Build history of the part. All positions in model axes, mm. Give positions to 0.01 mm unless a question says otherwise; leave off trailing zeros. Order: outer loops, then holes, each group sorted by start corner. A loop starts at its lowest first (then second) coordinate and runs counter-clockwise, first axis right, second up. Notation, with made-up numbers: (49, 12.5) - (74, 12.5) arc R12 ccw to (74, 16.5) - close; hole circle Ø10 at (-27, 24.25). An arc over 180 degrees is marked (long way). One line per item, written item: value.
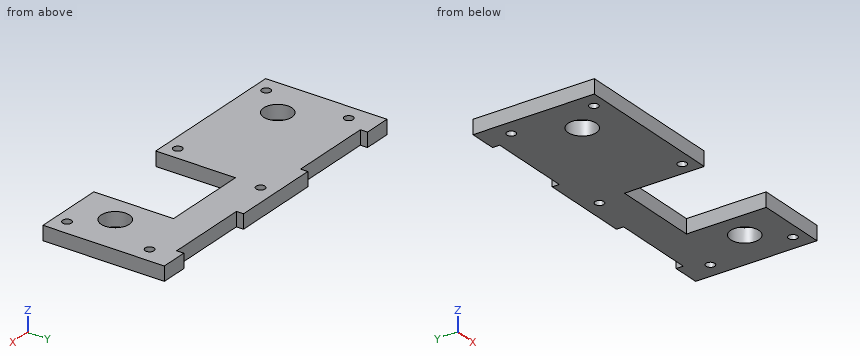
Autodesk Inventor part; units mm, degrees
ref_plane "YZ Plane" through (0, 0, 0) normal (1, 0, 0) x (0, 1, 0)
ref_plane "XZ Plane" through (0, 0, 0) normal (0, 1, 0) x (-1, 0, 0)
ref_plane "XY Plane" through (0, 0, 0) normal (0, 0, 1) x (1, 0, 0)
sketch "Boceto1" plane through (0, 0, 0) normal (0, 0, 1) x (1, 0, 0)
  arc A0 (-116.1173, -7.6512) -> (-117.6673, -9.2012) centre (-116.1173, -9.2012) ccw
  arc A1 (-117.6673, -9.2012) -> (-116.1173, -10.7512) centre (-116.1173, -9.2012) ccw
  arc A2 (-116.1173, -10.7512) -> (-114.5673, -9.2012) centre (-116.1173, -9.2012) ccw
  arc A3 (-114.5673, -9.2012) -> (-116.1173, -7.6512) centre (-116.1173, -9.2012) ccw
  arc A4 (-67.1173, -3.6512) -> (-68.6673, -5.2012) centre (-67.1173, -5.2012) ccw
  arc A5 (-68.6673, -5.2012) -> (-67.1173, -6.7512) centre (-67.1173, -5.2012) ccw
  arc A6 (-67.1173, -6.7512) -> (-65.5673, -5.2012) centre (-67.1173, -5.2012) ccw
  arc A7 (-65.5673, -5.2012) -> (-67.1173, -3.6512) centre (-67.1173, -5.2012) ccw
  arc A8 (-18.1173, -7.6512) -> (-19.6673, -9.2012) centre (-18.1173, -9.2012) ccw
  arc A9 (-19.6673, -9.2012) -> (-18.1173, -10.7512) centre (-18.1173, -9.2012) ccw
  arc A10 (-18.1173, -10.7512) -> (-16.5673, -9.2012) centre (-18.1173, -9.2012) ccw
  arc A11 (-16.5673, -9.2012) -> (-18.1173, -7.6512) centre (-18.1173, -9.2012) ccw
  arc A12 (-72.6173, -36.6512) -> (-74.1673, -38.2012) centre (-72.6173, -38.2012) ccw
  arc A13 (-74.1673, -38.2012) -> (-72.6173, -39.7512) centre (-72.6173, -38.2012) ccw
  arc A14 (-72.6173, -39.7512) -> (-71.0673, -38.2012) centre (-72.6173, -38.2012) ccw
  arc A15 (-71.0673, -38.2012) -> (-72.6173, -36.6512) centre (-72.6173, -38.2012) ccw
  arc A16 (-18.1173, -36.6512) -> (-19.6673, -38.2012) centre (-18.1173, -38.2012) ccw
  arc A17 (-19.6673, -38.2012) -> (-18.1173, -39.7512) centre (-18.1173, -38.2012) ccw
  arc A18 (-18.1173, -39.7512) -> (-16.5673, -38.2012) centre (-18.1173, -38.2012) ccw
  arc A19 (-16.5673, -38.2012) -> (-18.1173, -36.6512) centre (-18.1173, -38.2012) ccw
  arc A20 (-116.1173, -36.6512) -> (-117.6673, -38.2012) centre (-116.1173, -38.2012) ccw
  arc A21 (-117.6673, -38.2012) -> (-116.1173, -39.7512) centre (-116.1173, -38.2012) ccw
  arc A22 (-116.1173, -39.7512) -> (-114.5673, -38.2012) centre (-116.1173, -38.2012) ccw
  arc A23 (-114.5673, -38.2012) -> (-116.1173, -36.6512) centre (-116.1173, -38.2012) ccw
  arc A24 (-107.1173, -22.7512) -> (-112.0673, -27.7012) centre (-107.1173, -27.7012) ccw
  arc A25 (-112.0673, -27.7012) -> (-107.1173, -32.6512) centre (-107.1173, -27.7012) ccw
  arc A26 (-107.1173, -32.6512) -> (-102.1673, -27.7012) centre (-107.1173, -27.7012) ccw
  arc A27 (-102.1673, -27.7012) -> (-107.1173, -22.7512) centre (-107.1173, -27.7012) ccw
  arc A28 (-27.1173, -22.7512) -> (-32.0673, -27.7012) centre (-27.1173, -27.7012) ccw
  arc A29 (-32.0673, -27.7012) -> (-27.1173, -32.6512) centre (-27.1173, -27.7012) ccw
  arc A30 (-27.1173, -32.6512) -> (-22.1673, -27.7012) centre (-27.1173, -27.7012) ccw
  arc A31 (-22.1673, -27.7012) -> (-27.1173, -22.7512) centre (-27.1173, -27.7012) ccw
  line L0 (-67.8173, -14.5012) -> (-37.3173, -14.5012)
  line L1 (-37.3173, -14.5012) -> (-37.3173, -42.5012)
  line L2 (-37.3173, -42.5012) -> (-12.3173, -42.5012)
  line L3 (-12.3173, -42.5012) -> (-12.3173, 0.0988)
  line L4 (-12.3173, 0.0988) -> (-21.9173, 0.0988)
  line L5 (-21.9173, 0.0988) -> (-21.9173, -2.4012)
  line L6 (-21.9173, -2.4012) -> (-51.3173, -2.4012)
  line L7 (-51.3173, -2.4012) -> (-51.3173, 0.0988)
  line L8 (-51.3173, 0.0988) -> (-82.9173, 0.0988)
  line L9 (-82.9173, 0.0988) -> (-82.9173, -2.4012)
  line L10 (-82.9173, -2.4012) -> (-112.3173, -2.4012)
  line L11 (-112.3173, -2.4012) -> (-112.3173, 0.0988)
  line L12 (-112.3173, 0.0988) -> (-121.9173, 0.0988)
  line L13 (-121.9173, 0.0988) -> (-121.9173, -42.5012)
  line L14 (-121.9173, -42.5012) -> (-67.8173, -42.5012)
  line L15 (-67.8173, -42.5012) -> (-67.8173, -14.5012)
  point P0 (0, 0)
extrude "Extrusión1" add sketch "Boceto1" along normal blind 5
properties part number "carro x lado polea pieza2"
(1) Pin check, flat tips, straight feed: P1, Ø4, axis at x = -116.12, y = -38.2, coming from the +Z side; P2, Ø2.5, axis at x = -67.12, y = -5.2, coming from the +Z side. Stop position of each tip, or through.
Completed:
P1: z = 5
P2: through
(2) Slice it at A-A, the plane x = -30. Give the cut face in (y, z).
Completed:
outline: (-42.5, 0) - (-31.73, 0) - (-31.73, 5) - (-42.5, 5) - close; (-23.68, 0) - (-2.4, 0) - (-2.4, 5) - (-23.68, 5) - close
(3) Slice it at D-D, the plane x = -41. Give the cut face in (y, z).
Completed:
outline: (-14.5, 0) - (-2.4, 0) - (-2.4, 5) - (-14.5, 5) - close
(4) Drill centre lines: line 1 (X direction, y = -2, z = 1.9); line 2 (X direction, y = -27.5, z = 3.85); line 3 (X direction, y = -38, z = 1.6). Where is each one in solid material? Low to high.
Completed:
line 1: -121.92 to -112.32, -82.92 to -51.32, -21.92 to -12.32
line 2: -121.92 to -112.06, -102.17 to -67.82, -37.32 to -32.06, -22.17 to -12.32
line 3: -121.92 to -117.65, -114.58 to -74.15, -71.08 to -67.82, -37.32 to -19.65, -16.58 to -12.32
(5) Slice it at C-C, the plane z = 2.25. Count the separate pieces of the cut face and the enclosed holes in it, and give its area (3 significant figures).
Completed:
separate pieces: 1
enclosed holes: 8
area: 3,470 mm²
(6) Slice it at B-B, the plane y = -5. Give the cut face in (x, z), and give its area (3 significant figures).
Completed:
outline: (-121.92, 0) - (-68.65, 0) - (-68.65, 5) - (-121.92, 5) - close; (-65.58, 0) - (-12.32, 0) - (-12.32, 5) - (-65.58, 5) - close
area: 533 mm²
